Check sheet for the drawn part. Datum: minimum x, y, z corner. Units: mm. A direction names the side the tool comes from. Coordinates: 2 decimals unless noted, no trailing zeros. Loops run counter-clockwise (first coordinate to the right, second up) from the corner with the lowest first, then second, coordinate; pieces in that order, holes last.
Q1. Material ranges on probe 1 along Y at (x, z) = (37.5, 2.2); probe 2 along Z at (x, y) = (30, 7); probe 3 along Z at (x, y) = (8, 9.5), recorded low to high.
Q2. Go/stop test with flat-tipped pins: P1, Ø2, axis at y = 8, z = 4.5, coming from the +X side; P2, Ø5.5, axis at x = 24.5, z = 6, coming from the +Y side; P3, Ø2, axis at x = 21.5, y = 2.5, coming from the -Z side. Record where each tip stops, or that it passes through.
Q3. Sectioned sample at B-B (z = 4). Enter the section's corners in (x, y) (3 decimals).
Q4. Mould release check, pull along X, two halves, no side actions. Record for the marked faces 5, 6 and 7: +X half, -X half, draft (parallel to the pull), parting line (faces both ways), or undercut.
Q5. Sectioned sample at D-D (y = 10.25). Enter the section's corners in (x, z), then the cut area to 3 significant figures.
Q6. Sectioned sample at C-C (x = 29.5). Enter the section's corners in (y, z), then the cut area to 3 significant figures.
Q7. Sectioned sample at A-A (x = 7). Enter the section's corners in (y, z) (3 decimals).
Q8. Access from +Z, -Z, +X, -X, +Y, -Y to the whole of each face (thin tool, end or side, straight path). Record for the marked faces 1, 2, 3 and 4.
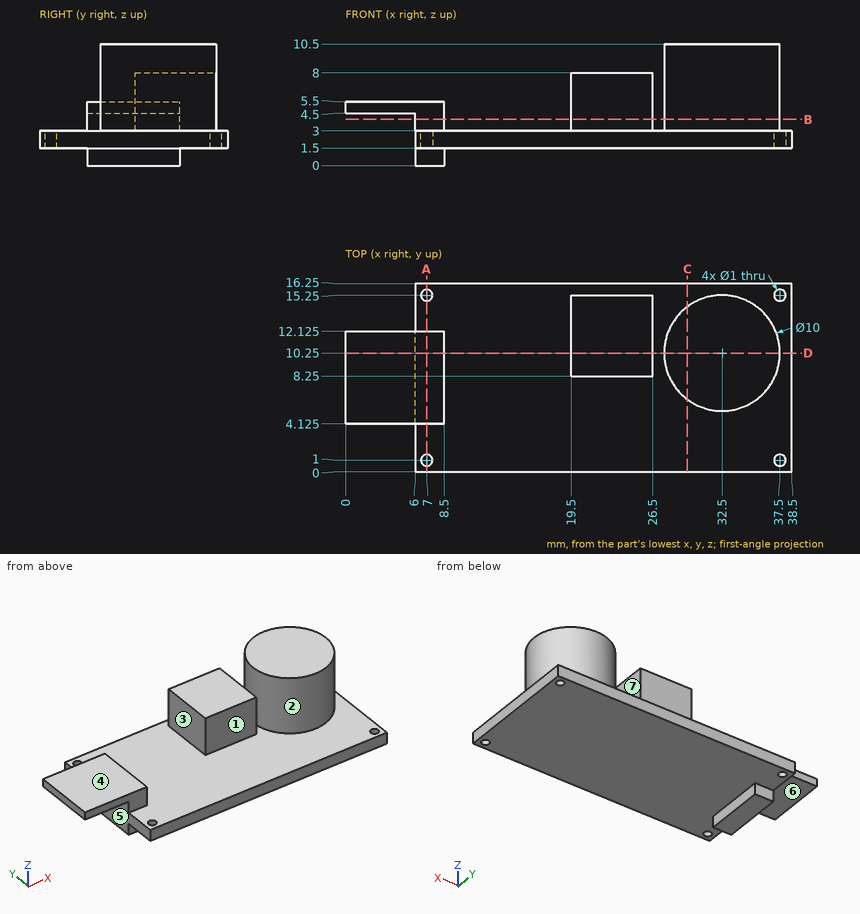
Geometry check:
1. probe 1: y = 0 to 0.5, 1.5 to 14.75, 15.75 to 16.25
1. probe 2: z = 1.5 to 10.5
1. probe 3: z = 0 to 5.5
2. P1: stops at x = 37.34
2. P2: stops at y = 15.25
2. P3: stops at z = 1.5
3. outline: (6, 4.125) - (8.5, 4.125) - (8.5, 12.125) - (6, 12.125) - close; (19.5, 8.25) - (26.5, 8.25) - (26.5, 15.25) - (19.5, 15.25) - close; circle Ø10 at (32.5, 10.25)
4. face 5: -X half
4. face 6: draft
4. face 7: undercut
5. outline: (0, 4.5) - (6, 4.5) - (6, 0) - (8.5, 0) - (8.5, 1.5) - (38.5, 1.5) - (38.5, 3) - (37.5, 3) - (37.5, 10.5) - (27.5, 10.5) - (27.5, 3) - (26.5, 3) - (26.5, 8) - (19.5, 8) - (19.5, 3) - (8.5, 3) - (8.5, 5.5) - (0, 5.5) - close
5. area: 175 mm2
6. outline: (0, 1.5) - (16.25, 1.5) - (16.25, 3) - (14.25, 3) - (14.25, 10.5) - (6.25, 10.5) - (6.25, 3) - (0, 3) - close
6. area: 84.4 mm2
7. outline: (0, 1.5) - (0.5, 1.5) - (0.5, 3) - (0, 3) - close; (1.5, 1.5) - (4.125, 1.5) - (4.125, 0) - (12.125, 0) - (12.125, 1.5) - (14.75, 1.5) - (14.75, 3) - (12.125, 3) - (12.125, 5.5) - (4.125, 5.5) - (4.125, 3) - (1.5, 3) - close; (15.75, 1.5) - (16.25, 1.5) - (16.25, 3) - (15.75, 3) - close
8. face 1: +Z, -Y
8. face 2: +Z
8. face 3: +Z, +Y, -Y
8. face 4: +Z, -X, +Y, -Y
